Work out the finished part from the listing and answer in its coordinate system (mm). A direction names the side the tool comes from. Coordinates: 2 decimals unless noted, no trailing zeros. Order: outer loops, then holes, each group sorted by start corner. A loop starts at its lowest first (then second) coordinate and runs counter-clockwise, first axis right, second up. Notation, with made-up numbers: M 67,79 L 82,79 A34 cw 82,115 Z; hole C 8.5,85.5 d5. An arc over 180 degrees is marked long. Write item = value, one per line. Start each with the question number.
Q1. Find section A-A on y = 3. Give the vertices of the cut face in (x, z), and give its area (3 significant figures).
Q2. Determine the mould class of faces 1 (the flat face through (-3, 12.5, 3)), 2 (the flat face through (0, 6, 200)), 3 (the cylindrical face through (-2.534, 9.813, 182.764)) for opening direction Z: released by +Z, released by -Z, zero draft, split by the parting line, or undercut.
Q3. Straight lines are drawn through the part: line 1 along Y through (x, z) = (-5.75, -49); line 2 along X through (y, z) = (2.75, -180); line 3 along X through (y, z) = (11.45, 60). For each, find the intervals that lie inside material, in ascending order.
Q4. A tool of negligible diameter and unlimited length cuts with its end or side. For faces 4 (the flat face through (-2, 7.2, -178)), 5 (the flat face through (0, 6, -200)), from which of +Z, -Z, +X, -X, +Y, -Y can it reach the whole face along a straight path? Write none if from no direction.
Q5. Each of these flat-tipped pins is pushed along its axis until it touches: P1, Ø7, axis at x = 0, z = 180, coming from the +Y side; P2, Ø0.5, axis at y = 8, z = -7.5, coming from the -X side. Where does it stop, or does it pass through?
Q6. Find section C-C on x = 0. Give the number of separate pieces and of enclosed holes in the cut face, and give its area (3 significant figures).
Q7. Find section B-B on z = 83. Give the vertices of the cut face in (x, y), and give its area (3 significant figures).
```python
from build123d import *

# Parameters (mm, degrees)
EXTRUDE1_DEPTH  = 200
LPATTERN1_COUNT = 6
LPATTERN1_PITCH = 60


with BuildPart() as part:
    # 15mm → Extrude1 (new, symmetric)
    with BuildSketch(Plane.XY):
        with BuildLine():
            Line((4.949972, 7.600006), (6.192321846, 7.599996))
            ThreePointArc((6.192321846, 7.599996), (6.706266371, 6.946742527), (7.49999, 6.7))
            Line((7.49999, 6.7), (7.49999, 1.000024142))
            Line((7.49999, 1.000024142), (6.499965858, 0))
            Line((6.499965858, 0), (-6.499965858, 0))
            Line((-6.499965858, 0), (-7.49999, 1.000024142))
            Line((-7.49999, 1.000024142), (-7.49999, 6.7))
            ThreePointArc((-7.49999, 6.7), (-6.70626637, 6.946742527), (-6.192321846, 7.599996))
            Line((-6.192321846, 7.599996), (-4.949982, 7.599996))
            Line((-4.949982, 7.599996), (-4.949972, 8.600006))
            Line((-4.949972, 8.600006), (-6.192326435, 8.600016))
            ThreePointArc((-6.192326435, 8.600016), (-6.706271662, 9.253261115), (-7.49999, 9.5))
            Line((-7.49999, 9.5), (-7.49999, 11.099974))
            ThreePointArc((-7.49999, 11.099974), (-6.510037425, 11.510033031), (-6.099989, 12.49999))
            Line((-6.099989, 12.49999), (6.099989, 12.49999))
            ThreePointArc((6.099989, 12.49999), (6.510037425, 11.510033031), (7.49999, 11.099974))
            Line((7.49999, 11.099974), (7.49999, 9.5))
            ThreePointArc((7.49999, 9.5), (6.706271662, 9.253261115), (6.192326435, 8.600016))
            Line((6.192326435, 8.600016), (4.949982, 8.600016))
            Line((4.949982, 8.600016), (4.949972, 7.600006))
        make_face()
    extrude(amount=EXTRUDE1_DEPTH, both=True)

    # Sketch1 → Cut-Revolve1 (revolve, cut)
    with BuildSketch(Plane(origin=(0, 0, 0), x_dir=(0, 0, -1), z_dir=(1, 0, 0))):
        Polygon((-180, 12.49999), (-176.25, 12.49999), (-176.25, 7.19999), (-177.75, 7.19999), (-177.75, 0), (-180, 0), align=None)
    revolve(axis=Axis((0, 0, 180), (0, 1, 0)), mode=Mode.SUBTRACT)

    # Sketch2 → Cut-Revolve2 (revolve, cut)
    with BuildSketch(Plane(origin=(0, 0, 0), x_dir=(0, 0, -1), z_dir=(1, 0, 0))):
        Polygon((180, 0), (182.25, 0), (182.25, 7.19999), (183.75, 7.19999), (183.75, 12.49999), (180, 12.49999), align=None)
    cut_revolve2 = revolve(axis=Axis((0, 12.49999, -180), (0, -1, 0)), mode=Mode.SUBTRACT)

    # LPattern1: Cut-Revolve2 ×6
    with Locations(*[(0, 0, i * LPATTERN1_PITCH) for i in range(1, LPATTERN1_COUNT)]):
        add(cut_revolve2, mode=Mode.SUBTRACT)


solid = part.part
```
Findings below:
q1.outline = M -7.5,-200 L 7.5,-200 L 7.5,200 L -7.5,200 Z; hole C 0,-180 d4.5; hole C 0,-120 d4.5; hole C 0,-60 d4.5; hole C 0,0 d4.5; hole C 0,60 d4.5; hole C 0,120 d4.5; hole C 0,180 d4.5
q1.area = 5,890 mm^2
q2.face_1 = zero draft
q2.face_2 = released by +Z
q2.face_3 = undercut
q3.line_1 = 0 to 7.6, 8.6 to 12.5
q3.line_2 = -7.5 to -2.25, 2.25 to 7.5
q3.line_3 = -6.57 to -3.75, 3.75 to 6.57
q4.face_4 = +Y
q4.face_5 = -Z, +X, -X, +Y, -Y
q5.P1 = 7.2
q5.P2 = -4.95
q6.separate_pieces = 8
q6.enclosed_holes = 0
q6.area = 4,490 mm^2
q7.outline = M -7.5,1 L -6.5,0 L 6.5,0 L 7.5,1 L 7.5,6.7 A1.4 cw 6.19,7.6 L 4.95,7.6 L 4.95,8.6 L 6.19,8.6 A1.4 cw 7.5,9.5 L 7.5,11.1 A1.4 cw 6.1,12.5 L -6.1,12.5 A1.4 cw -7.5,11.1 L -7.5,9.5 A1.4 cw -6.19,8.6 L -4.95,8.6 L -4.95,7.6 L -6.19,7.6 A1.4 cw -7.5,6.7 Z
q7.area = 175 mm^2
